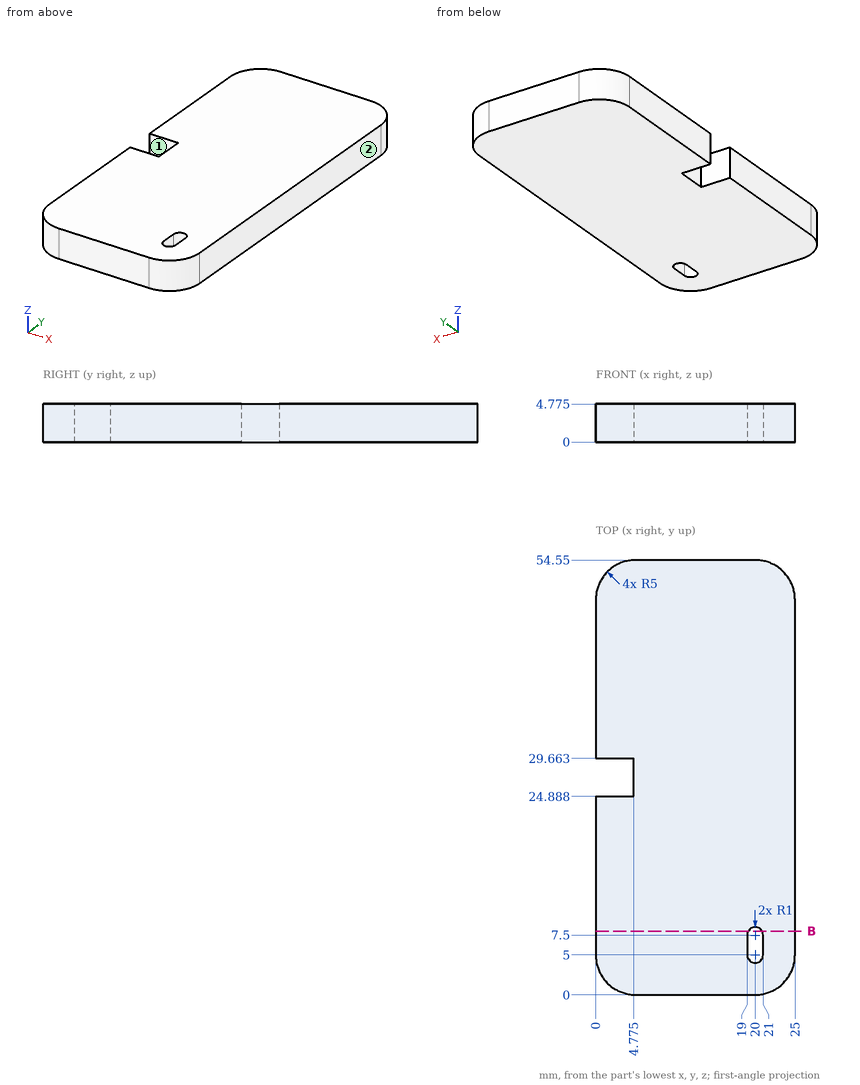
Could you check a few things on this drawing? It's one solid part, dimensions in mm from its lowest x, y, z. A direction names the side the tool comes from. Give positions to 0.01 mm unless a question says otherwise; leave off trailing zeros. Write each loop counter-clockwise with the first axis right and the second up, starting at its lowest first coordinate (ties: lowest second). Pieces come first, ordered by that corner, then holes. Notation, with made-up numbers: (16, -25.75) -> (48, -25.75) arc R32 ccw to (48, 4.25) -> close; hole circle Ø9 at (81.25, 19.5). An arc over 180 degrees is marked (long way). Write item = value, one per line.
(1) For the marked faces 1 and 2, which set-ups out of +Z, -Z, +X, -X, +Y, -Y let a thin tool reach every point of the face, with its end or its side?
Worked out:
face_1 = +Z, -Z, -X
face_2 = +Z, -Z, +X, +Y, -Y
(2) I'm going to push flat-ended pins straight in: P1, Ø2.5, axis at x = 3, z = 2, coming from the +Y side; P2, Ø3, axis at x = 4, y = 44.5, coming from the -Z side. Where does each tip first touch, or does it pass through?
Worked out:
P1 = 54.49
P2 = 0
(3) Suppose I cut it at B-B on y = 8. Write out the boundary of the cut face in (x, z) (1 decimal).
Worked out:
outline = (0, 0) -> (19.1, 0) -> (19.1, 4.8) -> (0, 4.8) -> close; (20.9, 0) -> (25, 0) -> (25, 4.8) -> (20.9, 4.8) -> close
(4) I need wall thicknesses on probe 1 along Y at (x, z) = (20, 1.45); probe 2 along X at (y, z) = (26, 2.1) (1 decimal); probe 3 along Y at (x, z) = (3.5, 0.4). Which ranges of each line are inside material? Lowest first, please. Write a range as from..to.
Worked out:
probe_1 = 0..4, 8.5..54.55
probe_2 = 4.8..25
probe_3 = 0.23..24.89, 29.66..54.32
